from build123d import *

# Parameters (mm, degrees)
BOSS_EXTRUDE1_DEPTH = 6.35
SKETCH2_R           = 5.08
CUT_EXTRUDE1_DEPTH  = 201.754423986
SKETCH3_R           = 2.159
CUT_EXTRUDE2_DEPTH  = 201.754423986
SKETCH4_R           = 3.175
CUT_EXTRUDE3_DEPTH  = 201.754423986
SKETCH6_R           = 2.159
CUT_EXTRUDE5_DEPTH  = 201.754423986


with BuildPart() as part:
    # Sketch1 → Boss-Extrude1 (new body)
    with BuildSketch(Plane(origin=(0, 0, 0), x_dir=(1, 0, 0), z_dir=(0, 1, 0))):
        with BuildLine():
            Line((-174.625, 12.7), (174.625, 12.7))
            ThreePointArc((174.625, 12.7), (200.025, 0), (174.625, -12.7))
            Line((174.625, -12.7), (-174.625, -12.7))
            ThreePointArc((-174.625, -12.7), (-200.025, 0), (-174.625, 12.7))
        make_face()
    extrude(amount=BOSS_EXTRUDE1_DEPTH)

    # Sketch2 → Cut-Extrude1 (cut, through all)
    with BuildSketch(Plane(origin=(0, 6.35, 0), x_dir=(1, 0, 0), z_dir=(0, 1, 0))):
        with Locations(Location((184.15, 0, 0), (0, 0, 270))):
            Circle(SKETCH2_R)
        with Locations(Location((-184.15, 0, 0), (0, 0, 90))):
            Circle(SKETCH2_R)
        with BuildLine():
            Line((173.691383345, 1.25), (175.608616655, 1.25))
            ThreePointArc((175.608616655, 1.25), (176.858616655, 0), (175.608616655, -1.25))
            Line((175.608616655, -1.25), (173.691383345, -1.25))
            ThreePointArc((173.691383345, -1.25), (172.441383345, 0), (173.691383345, 1.25))
        make_face()
        with BuildLine():
            Line((194.608616655, 1.25), (192.691383345, 1.25))
            ThreePointArc((192.691383345, 1.25), (191.441383345, 0), (192.691383345, -1.25))
            Line((192.691383345, -1.25), (194.608616655, -1.25))
            ThreePointArc((194.608616655, -1.25), (195.858616655, 0), (194.608616655, 1.25))
        make_face()
        with BuildLine():
            Line((185.4, 8.920928665), (185.4, 6.921035691))
            ThreePointArc((185.4, 6.921035691), (184.15, 5.671035691), (182.9, 6.921035691))
            Line((182.9, 6.921035691), (182.9, 8.920928665))
            ThreePointArc((182.9, 8.920928665), (184.15, 10.170928665), (185.4, 8.920928665))
        make_face()
        with BuildLine():
            Line((185.441381345, -9.078964309), (185.441381345, -7.078964309))
            ThreePointArc((185.441381345, -7.078964309), (184.191381345, -5.828964309), (182.941381345, -7.078964309))
            Line((182.941381345, -7.078964309), (182.941381345, -9.078964309))
            ThreePointArc((182.941381345, -9.078964309), (184.191381345, -10.328964309), (185.441381345, -9.078964309))
        make_face()
        with BuildLine():
            Line((-185.441381345, -9.078964309), (-185.441381345, -7.078964309))
            ThreePointArc((-185.441381345, -7.078964309), (-184.191381345, -5.828964309), (-182.941381345, -7.078964309))
            Line((-182.941381345, -7.078964309), (-182.941381345, -9.078964309))
            ThreePointArc((-182.941381345, -9.078964309), (-184.191381345, -10.328964309), (-185.441381345, -9.078964309))
        make_face()
        with BuildLine():
            Line((-185.4, 8.920928665), (-185.4, 6.921035691))
            ThreePointArc((-185.4, 6.921035691), (-184.15, 5.671035691), (-182.9, 6.921035691))
            Line((-182.9, 6.921035691), (-182.9, 8.920928665))
            ThreePointArc((-182.9, 8.920928665), (-184.15, 10.170928665), (-185.4, 8.920928665))
        make_face()
        with BuildLine():
            Line((-194.608616655, 1.25), (-192.691383345, 1.25))
            ThreePointArc((-192.691383345, 1.25), (-191.441383345, 0), (-192.691383345, -1.25))
            Line((-192.691383345, -1.25), (-194.608616655, -1.25))
            ThreePointArc((-194.608616655, -1.25), (-195.858616655, 0), (-194.608616655, 1.25))
        make_face()
        with BuildLine():
            Line((-173.691383345, 1.25), (-175.608616655, 1.25))
            ThreePointArc((-175.608616655, 1.25), (-176.858616655, 0), (-175.608616655, -1.25))
            Line((-175.608616655, -1.25), (-173.691383345, -1.25))
            ThreePointArc((-173.691383345, -1.25), (-172.441383345, 0), (-173.691383345, 1.25))
        make_face()
    extrude(amount=-CUT_EXTRUDE1_DEPTH, mode=Mode.SUBTRACT)

    # Sketch3 → Cut-Extrude2 (cut, through all)
    with BuildSketch(Plane(origin=(0, 6.35, 0), x_dir=(1, 0, 0), z_dir=(0, 1, 0))):
        with Locations(Location((0, 0, 0), (0, 0, 270))):
            Circle(SKETCH3_R)
        with Locations(Location((38.1, 0, 0), (0, 0, 270))):
            Circle(SKETCH3_R)
        with Locations(Location((-38.1, 0, 0), (0, 0, 270))):
            Circle(SKETCH3_R)
    extrude(amount=-CUT_EXTRUDE2_DEPTH, mode=Mode.SUBTRACT)

    # Sketch4 → Cut-Extrude3 (cut, through all)
    with BuildSketch(Plane(origin=(0, 6.35, 0), x_dir=(1, 0, 0), z_dir=(0, 1, 0))):
        with Locations(Location((-19.05, 0, 0), (0, 0, 270))):
            Circle(SKETCH4_R)
        with Locations(Location((19.05, 0, 0), (0, 0, 270))):
            Circle(SKETCH4_R)
    extrude(amount=-CUT_EXTRUDE3_DEPTH, mode=Mode.SUBTRACT)

    # Sketch6 → Cut-Extrude5 (cut, through all)
    with BuildSketch(Plane(origin=(0, 0, 0), x_dir=(-1, 0, 0), z_dir=(0, -1, 0))):
        with Locations(Location((54.61, 1.2e-08, 0), (0, 0, 90))):
            Circle(SKETCH6_R)
        with Locations(Location((-54.61, 0, 0), (0, 0, 90))):
            Circle(SKETCH6_R)
    extrude(amount=-CUT_EXTRUDE5_DEPTH, mode=Mode.SUBTRACT)


solid = part.part
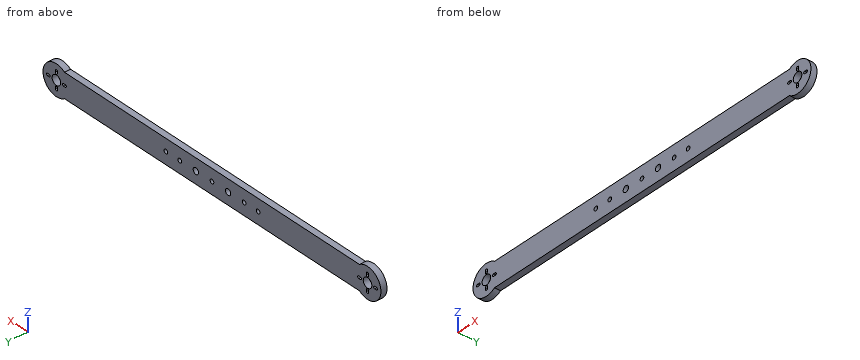
Here's how the part is built. I have some questions about the finished solid (model axes, mm). Coordinates: 2 decimals unless noted, no trailing zeros. Order: outer loops, then holes, each group sorted by start corner. A loop starts at its lowest first (then second) coordinate and runs counter-clockwise, first axis right, second up. Notation, with made-up numbers: M 40,50 L 52,50 A25 cw 52,70 Z; hole C 85.5,-8.75 d5. An arc over 180 degrees is marked long. Answer as CSV lines item,"result".
Item 1: If I drill on line 1 (Z direction, x = -184.15, y = 1.5) (3 decimals); line 2 (X direction, y = 3.5, z = 9.5); line 3 (X direction, y = 4.75, z = 14.5), over which ranges is the centre line in solid material (lowest first)?
Results found:
line 1,"-15.875 to -10.171, -5.671 to -5.08, 5.08 to 5.83, 10.328 to 15.875"
line 2,"-196.87 to -185.37, -183.01 to 183.01, 185.37 to 196.87"
line 3,"-190.61 to -177.69, 177.69 to 190.61"
Item 2: Imagine slicing it at B-B on x = -75.5. Write out the boundary of the cut face in (y, z).
Results found:
outline,"M 0,-12.7 L 6.35,-12.7 L 6.35,12.7 L 0,12.7 Z"
Item 3: For pin 1 (2 mm diameter, centred on x = -194, y = 3, fed in from -Z); pin 2 (3 mm diameter, centred on x = -1.5, y = 5.5, fed in from -Z); pin 3 (1 mm diameter, centred on x = -175, y = 4, fed in from +Z); pin 4 (8.5 mm diameter, centred on x = -19.05, z = 0, fed in from +Y), each with a flat end and sliding along its axis, tell me the tip position at first contact or that it passes through.
Results found:
pin 1,"z = -13.18"
pin 2,"z = -12.7"
pin 3,"z = 13.31"
pin 4,"y = 6.35"
Item 4: Imagine slicing it at A-A on y = 4.25. Give the number of separate pieces and of enclosed holes in the cut face, plus the area to 3 significant figures.
Results found:
separate pieces,"1"
enclosed holes,"17"
area,"9,850 mm2"
